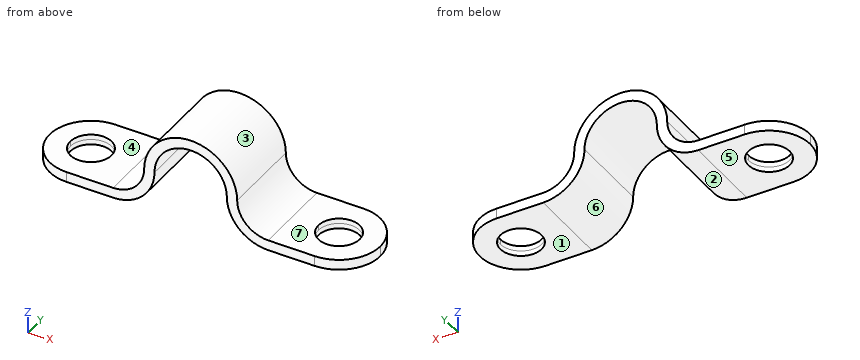
```python
from build123d import *

# Parameters (mm, degrees)
F1_DEPTH = 6.35
F2_R     = 6.34999
F4_D     = 6.35
F4_DEPTH = 12.701
F5_D     = 6.35


# Not quite as in the source:
# - a fillet or chamfer is up to 0.001 mm smaller than in the source, because OpenCascade refuses the exact size


with BuildPart() as f1:
    # F0 (on Front) → F1 (new body, symmetric)
    with BuildSketch(Plane.XZ):
        with BuildLine():
            Line((-11.90625, 0.79375), (-25.4, 0.79375))
            Line((-25.4, 0.79375), (-25.4, -0.79375))
            Line((-25.4, -0.79375), (-11.90625, -0.79375))
            ThreePointArc((-11.90625, -0.79375), (-7.4161219395, 1.0661219395), (-5.55625, 5.55625))
            ThreePointArc((-5.55625, 5.55625), (0, 11.1125), (5.55625, 5.55625))
            ThreePointArc((5.55625, 5.55625), (7.4161219395, 1.0661219395), (11.90625, -0.79375))
            Line((11.90625, -0.79375), (25.4, -0.79375))
            Line((25.4, -0.79375), (25.4, 0.79375))
            Line((25.4, 0.79375), (11.90625, 0.79375))
            ThreePointArc((11.90625, 0.79375), (8.5386539546, 2.1886539546), (7.14375, 5.55625))
            ThreePointArc((7.14375, 5.55625), (0, 12.7), (-7.14375, 5.55625))
            ThreePointArc((-7.14375, 5.55625), (-8.5386539546, 2.1886539546), (-11.90625, 0.79375))
        make_face()
    extrude(amount=F1_DEPTH, both=True)

    # F2 (radius 6.35 in the source; OpenCascade refuses exactly that, so slightly less here)
    f2_edges = [f1.edges().sort_by_distance(p)[0] for p in [
        (25.4, -6.35, 0),
        (25.4, 6.35, 0),
        (-25.4, -6.35, 0),
        (-25.4, 6.35, 0),
    ]]
    fillet(f2_edges, radius=F2_R)

    # F4 (through all, one way)
    with BuildSketch(Plane(origin=(0, 0, 0), x_dir=(1, 0, 0), z_dir=(0, 0, -1))):
        with Locations((-19.05, 0), (19.05, 0)):
            Circle(F4_D / 2)
    extrude(amount=-F4_DEPTH, mode=Mode.SUBTRACT)

    # F5 (through all)
    with Locations(Plane.XY):
        with Locations((-19.05, 0), (19.05, 0)):
            Hole(F5_D / 2)


solid = f1.part
```
Model file for the job. Use its own axes, mm. Face numbers are marked on the shaded views. A direction names the side the tool comes from. Give positions to 0.01 mm unless a question says otherwise; leave off trailing zeros. Write each loop counter-clockwise with the first axis right and the second up, starting at its lowest first coordinate (ties: lowest second). Pieces come first, ordered by that corner, then holes. Notation, with made-up numbers: M -6,70 L 48,70 A26 ccw 48,90 Z; hole C 53,-7 d8. An arc over 180 degrees is marked long. Use a Markdown table: item, result.
1) Drill centre lines: line 1 (Y direction, x = -19.05, z = -0.35) (3 decimals); line 2 (X direction, y = 0, z = -0.25) (3 decimals); line 3 (X direction, y = 0.5, z = 2). Where is each one in solid material? Low to high. Write a range as from..to.
Responses:
| item | result |
|---|---|
| line 1 | y = -6.35..-3.175, 3.175..6.35 |
| line 2 | x = -25.4..-22.225, -15.875..-9.335, 9.335..15.875, 22.225..25.4 |
| line 3 | x = -8.74..-6.65, 6.65..8.74 |
2) Cut at B-B (z = 7.75). List the corners of the cut face in (x, y), and give its area (3 significant figures).
Responses:
| item | result |
|---|---|
| outline | M -6.8,-6.35 L -5.1,-6.35 L -5.1,6.35 L -6.8,6.35 Z; M 5.1,-6.35 L 6.8,-6.35 L 6.8,6.35 L 5.1,6.35 Z |
| area | 43.0 mm2 |
3) Cut at A-A (y = 0.75). Give the number of separate pieces and of enclosed holes in the cut face, and give its area (3 significant figures).
Responses:
| item | result |
|---|---|
| separate pieces | 3 |
| enclosed holes | 0 |
| area | 82.5 mm2 |
4) Tool access for the marked faces 4, 5, 6 and 7: list every direction of +Z, -Z, +X, -X, +Y, -Y with a clear straight run to the whole face (end or side of a thin tool).
Responses:
| item | result |
|---|---|
| face 4 | +Z, -X, +Y, -Y |
| face 5 | -Z, +X, -X, +Y, -Y |
| face 6 | -Z, +Y, -Y |
| face 7 | +Z, +X, +Y, -Y |
5) Pin check, flat tips, straight feed: pin 1 (1.5 mm diameter, centred on x = -5, y = -3.5, fed in from +Z); pin 2 (5 mm diameter, centred on x = -19.05, y = 0, fed in from -Z); pin 3 (2 mm diameter, centred on y = 4.5, z = 6, fed in from -X); pin 4 (2 mm diameter, centred on y = 4, z = 1.5, fed in from +X). Stop position of each tip, or through.
Responses:
| item | result |
|---|---|
| pin 1 | stops at z = 11.3 |
| pin 2 | passes through |
| pin 3 | stops at x = -7.18 |
| pin 4 | stops at x = 24.48 |
6) Pull direction X, two halves, no side cores. Call the marked faces 1, 2 and 3: +X half, -X half, draft (parallel to the pull), parting line (faces both ways), or undercut.
Responses:
| item | result |
|---|---|
| face 1 | draft |
| face 2 | undercut |
| face 3 | parting line |
7) Cut at C-C (x = 18.5). List the corners of the cut face in (y, z).
Responses:
| item | result |
|---|---|
| outline | M -6.35,-0.79 L -3.13,-0.79 L -3.13,0.79 L -6.35,0.79 Z; M 3.13,-0.79 L 6.35,-0.79 L 6.35,0.79 L 3.13,0.79 Z |
